For this review, take the finished solid that the model builds, in its own axes (mm). A direction names the side the tool comes from. Round coordinates to 2 decimals unless told otherwise and drop trailing zeros. Write each loop counter-clockwise with the first axis right and the second up, starting at its lowest first coordinate (ties: lowest second). Pieces come first, ordered by that corner, then holes. Notation, with made-up numbers: (16.25, 62.25) - (22.25, 62.25) arc R12 cw to (22.25, 76.25) - close; hole circle Ø6 at (-2, 77.25). An arc over 180 degrees is marked (long way). One line per item, written item: value. Start each with the question number.
Q1. Mouldability with a two-part tool opening along Y and no side actions: class faces 6 (the face through (711, 25.082, 6)), 7 (the face through (797.043, 30.166, 5.54)), 8 (the face through (712, 33.338, 4)) as +Y half, -Y half, draft (parallel to the pull), parting line (faces both ways), or undercut.
Q2. Add section B-B on x = 727.5. Write out the cut boundary in (y, z).
Q3. Add section A-A on y = -9.5. Write out the cut boundary in (x, z) (3 decimals), and give its area (3 significant figures).
Q4. Add section D-D on x = 772. Write out the cut boundary in (y, z), and give its area (3 significant figures).
Q5. Add section C-C on z = 9.5. Give the number of separate pieces and of enclosed holes in the cut face, and give its area (3 significant figures).
Q6. For probe 1 along Y at (x, z) = (793, 6.5); probe 2 along Y at (x, z) = (752, 1.5); probe 3 along X at (y, z) = (-28, 8.75), list the stretches that pass through material, from the lowest coordinate up.
Q7. Clearance check with flat-ended pins moving along their axes: pin 1 Ø0.6 at (y, z) = (-10, 1) entering from -X; pin 2 Ø2 at (x, z) = (768, 1) entering from -Y; pin 3 Ø10 at (x, y) = (772, -11) entering from -Z; pin 4 Ø0.6 at (y, z) = (7, 0.5) entering from +X (3 decimals). State where each tip first meets the part, or that it passes through.
Q8. Tool access review of faces 1 (the face through (789.37, 1, 1)), 2 (the face through (729.045, 29, 1)), 3 (the face through (784.29, -29, 5)), 4 (the face through (721.71, -23, 3)), 5 (the face through (713, -23, 7)): name each direction out of +Z, -Z, +X, -X, +Y, -Y from which nothing blocks a thin tool from reaching the whole face with its end or side.
```python
from build123d import *

# Parameters (mm, degrees)
EXTRUDE_1_DEPTH             = 8.255
EXTRUDE_2_DEPTH             = 50.165
CUT_EXTRUDE_1_DEPTH         = 50.165
EXTRUDE_3_DEPTH             = 8.255
CUT_EXTRUDE_2_DEPTH         = 8.255
CUT_EXTRUDE_3_DEPTH         = 8.255
CUT_EXTRUDE_4_DEPTH         = 55.245
CUT_EXTRUDE_5_DEPTH         = 0.635
CUT_EXTRUDE_6_DEPTH         = 46.99
SKETCH_10_W                 = 8.255
SKETCH_10_H                 = 4
EXTRUDE_4_DEPTH             = 0.635
CUT_EXTRUDE_7_DEPTH         = 2
EXTRUDE_5_DEPTH             = 8.255
SKETCH_13_W                 = 11.176
SKETCH_13_H                 = 4.318
CUT_EXTRUDE_8_DEPTH         = 3
CUT_EXTRUDE_9_DEPTH         = 12
SKETCH_15_W                 = 7.62
SKETCH_15_H                 = 31.75
CUT_EXTRUDE_10_DEPTH        = 3
HOLE_WIZARD_3_6_3_6_1_D     = 3.6
HOLE_WIZARD_3_6_3_6_1_DEPTH = 11
HOLE_WIZARD_3_6_3_6_2_D     = 3.6
HOLE_WIZARD_3_6_3_6_2_DEPTH = 11
FILLET_1_R                  = 0.635
FILLET_2_R                  = 2


with BuildPart() as part:
    # 草图1 → 凸台-拉伸1 (new body)
    with BuildSketch(Plane.XZ.offset(-25.0825)):
        with BuildLine():
            Line((729.045, 11), (729.045, 4))
            Line((729.045, 4), (721.71, 4))
            Line((721.71, 4), (718.71, 7))
            Line((718.71, 7), (715.71, 7))
            Line((715.71, 7), (715.71, 11))
            Line((715.71, 11), (705.298322179, 11))
            ThreePointArc((705.298322179, 11), (702.984819943, 5.616840019), (701.316943399, 0))
            Line((701.316943399, 0), (798.683056601, 0))
            ThreePointArc((798.683056601, 0), (797.015180057, 5.616840019), (794.701677821, 11))
            Line((794.701677821, 11), (729.045, 11))
        make_face()
    extrude(amount=-EXTRUDE_1_DEPTH)

    # 草图2 → 凸台-拉伸2 (add)
    with BuildSketch(Plane.XZ.offset(-25.0825)):
        with BuildLine():
            Line((705.298322179, 11), (715.71, 11))
            Line((715.71, 11), (715.71, 7))
            Line((715.71, 7), (718.71, 7))
            Line((718.71, 7), (721.71, 4))
            Line((721.71, 4), (792.545, 4))
            Line((792.545, 4), (792.545, 0))
            Line((792.545, 0), (701.316943399, 0))
            ThreePointArc((701.316943399, 0), (702.984819943, 5.616840019), (705.298322179, 11))
        make_face()
    extrude(amount=EXTRUDE_2_DEPTH)

    # 草图3 → 切除-拉伸1 (cut)
    with BuildSketch(Plane.XZ.offset(25.0825)):
        with BuildLine():
            Line((701.316943399, 0), (707.455, 0))
            Line((707.455, 0), (707.455, 7))
            Line((707.455, 7), (715.71, 7))
            Line((715.71, 7), (715.71, 11))
            Line((715.71, 11), (705.298322179, 11))
            ThreePointArc((705.298322179, 11), (702.984819943, 5.616840019), (701.316943399, 0))
        make_face()
    extrude(amount=-CUT_EXTRUDE_1_DEPTH, mode=Mode.SUBTRACT)

    # 草图4 → 凸台-拉伸3 (add)
    with BuildSketch(Plane.XZ.offset(25.0825)):
        with BuildLine():
            Line((705.298322179, 11), (715.71, 11))
            Line((715.71, 11), (715.71, 7))
            Line((715.71, 7), (718.71, 7))
            Line((718.71, 7), (721.71, 4))
            Line((721.71, 4), (792.545, 4))
            Line((792.545, 4), (792.545, 0))
            Line((792.545, 0), (701.316943399, 0))
            ThreePointArc((701.316943399, 0), (702.984819943, 5.616840019), (705.298322179, 11))
        make_face()
    extrude(amount=EXTRUDE_3_DEPTH)

    # 草图5 → 切除-拉伸2 (cut)
    with BuildSketch(Plane(origin=(0, 33.3375, 0), x_dir=(-1, 0, 0), z_dir=(0, 1, 0))):
        Polygon((-721.71, 4), (-715.71, 4), (-715.71, 7), (-718.71, 7), align=None)
    extrude(amount=-CUT_EXTRUDE_2_DEPTH, mode=Mode.SUBTRACT)

    # 草图6 → 切除-拉伸3 (cut)
    with BuildSketch(Plane.XZ.offset(33.3375)):
        Polygon((715.71, 0), (792.545, 0), (792.545, 4), (721.71, 4), (718.71, 7), (715.71, 7), align=None)
    extrude(amount=-CUT_EXTRUDE_3_DEPTH, mode=Mode.SUBTRACT)

    # 草图7 → 切除-拉伸4 (cut)
    with BuildSketch(Plane.ZY.offset(-729.045)):
        Polygon((0, 33.3375), (0, 24.8705), (4, 24.8705), (4, 25.0825), (11, 25.0825), (11, 33.3375), align=None)
    extrude(amount=-CUT_EXTRUDE_4_DEPTH, mode=Mode.SUBTRACT)

    # 草图8 → 切除-拉伸5 (cut)
    with BuildSketch(Plane.XZ.offset(25.0825)):
        Polygon((715.71, 0), (792.545, 0), (792.545, 4), (721.71, 4), (718.71, 7), (715.71, 7), align=None)
    extrude(amount=-CUT_EXTRUDE_5_DEPTH, mode=Mode.SUBTRACT)

    # 草图9 → 切除-拉伸6 (cut)
    with BuildSketch(Plane(origin=(0, 25.0825, 0), x_dir=(-1, 0, 0), z_dir=(0, 1, 0))):
        Polygon((-721.71, 4), (-714.44, 4), (-714.44, 0), (-707.455, 0), (-707.455, 7), (-718.71, 7), align=None)
    extrude(amount=-CUT_EXTRUDE_6_DEPTH, mode=Mode.SUBTRACT)

    # 草图10 → 凸台-拉伸4 (add)
    with BuildSketch(Plane.XZ.offset(24.4475)):
        with Locations((788.4175, 2)):
            Rectangle(SKETCH_10_W, SKETCH_10_H)
    extrude(amount=EXTRUDE_4_DEPTH)

    # 草图11 → 切除-拉伸7 (cut)
    with BuildSketch(Plane.XY.offset(4)):
        Polygon((784.29, 25.0825), (784.29, 24.8705), (729.045, 24.8705), (729.045, 33.3375), (715.71, 33.3375), (715.71, 25.0825), (714.44, 25.0825), (714.44, -21.9075), (721.71, -21.9075), (721.71, -24.4475), (784.29, -24.4475), (784.29, -25.0825), (792.545, -25.0825), (792.545, 25.0825), align=None)
    extrude(amount=-CUT_EXTRUDE_7_DEPTH, mode=Mode.SUBTRACT)

    # 草图12 → 凸台-拉伸5 (add)
    with BuildSketch(Plane.XZ.offset(25.0825)):
        with BuildLine():
            Line((798.683056601, 0), (784.29, 0))
            Line((784.29, 0), (784.29, 11))
            Line((784.29, 11), (794.701677821, 11))
            ThreePointArc((794.701677821, 11), (797.015180057, 5.616840019), (798.683056601, 0))
        make_face()
    extrude(amount=EXTRUDE_5_DEPTH)

    # 草图13 → 切除-拉伸8 (cut, through all)
    with BuildSketch(Plane.XY.offset(2)):
        with Locations((739.713, -22.2885)):
            Rectangle(SKETCH_13_W, SKETCH_13_H)
    extrude(amount=-CUT_EXTRUDE_8_DEPTH, mode=Mode.SUBTRACT)

    # 草图14 → 切除-拉伸9 (cut, through all)
    with BuildSketch(Plane(origin=(0, 0, 0), x_dir=(-1, 0, 0), z_dir=(0, 0, -1))):
        with BuildLine():
            Line((-777.963, 18.3705), (-777.963, 1.3705))
            Line((-777.963, 1.3705), (-778.963, 1.3705))
            Line((-778.963, 1.3705), (-778.963, -5.6295))
            Line((-778.963, -5.6295), (-777.963, -5.6295))
            Line((-777.963, -5.6295), (-777.963, -13.6295))
            ThreePointArc((-777.963, -13.6295), (-775.488126266, -14.654626266), (-774.463, -17.1295))
            Line((-774.463, -17.1295), (-724.463, -17.1295))
            ThreePointArc((-724.463, -17.1295), (-723.437873734, -14.654626266), (-720.963, -13.6295))
            Line((-720.963, -13.6295), (-720.963, 18.3705))
            ThreePointArc((-720.963, 18.3705), (-723.437873734, 19.395626266), (-724.463, 21.8705))
            Line((-724.463, 21.8705), (-774.463, 21.8705))
            ThreePointArc((-774.463, 21.8705), (-775.488126266, 19.395626266), (-777.963, 18.3705))
        make_face()
    extrude(amount=-CUT_EXTRUDE_9_DEPTH, mode=Mode.SUBTRACT)

    # 草图15 → 切除-拉伸10 (cut, through all)
    with BuildSketch(Plane.XY.offset(2)):
        with Locations((785.56, 0.9525)):
            Rectangle(SKETCH_15_W, SKETCH_15_H)
    extrude(amount=-CUT_EXTRUDE_10_DEPTH, mode=Mode.SUBTRACT)

    # Ø3.6 (3.6) 直径孔1
    with Locations(Plane(origin=(0, 0, 0), x_dir=(-1, 0, 0), z_dir=(0, 0, -1))):
        with Locations((-711.265, 29.5275), (-788.735, 29.5275), (-788.735, -29.5275), (-711.265, -29.5275)):
            Hole(HOLE_WIZARD_3_6_3_6_1_D / 2, depth=HOLE_WIZARD_3_6_3_6_1_DEPTH)

    # Ø3.6 (3.6) 直径孔2
    with Locations(Plane(origin=(0, 0, 0), x_dir=(-1, 0, 0), z_dir=(0, 0, -1))):
        with Locations((-720.963, -17.1295), (-720.963, 21.8705), (-777.963, 21.8705), (-777.963, -17.1295)):
            Hole(HOLE_WIZARD_3_6_3_6_2_D / 2, depth=HOLE_WIZARD_3_6_3_6_2_DEPTH)

    # 圆角1
    fillet_1_edges = [part.edges().sort_by_distance(p)[0] for p in [
        (711.5825, -25.0825, 7),
        (707.455, -23.495, 7),
        (707.455, -25.0825, 3.5),
    ]]
    fillet(fillet_1_edges, radius=FILLET_1_R)

    # 圆角2
    fillet_2_edges = [part.edges().sort_by_distance(p)[0] for p in [
        (797.015180057, -25.0825, 5.616840019),
        (702.984819943, 25.0825, 5.616840019),
        (702.984819943, -25.0825, 5.616840019),
        (797.015180057, 25.0825, 5.616840019),
    ]]
    fillet(fillet_2_edges, radius=FILLET_2_R)


solid = part.part
```
Result set:
1. face 6: undercut
1. face 7: draft
1. face 8: +Y half
2. outline: (-24.45, 0) - (-17.13, 0) - (-17.13, 2) - (-24.45, 2) - close; (21.87, 0) - (33.34, 0) - (33.34, 2) - (21.87, 2) - close
3. outline: (714.44, 0) - (720.963, 0) - (720.963, 2) - (714.44, 2) - close; (777.963, 0) - (781.75, 0) - (781.75, 2) - (777.963, 2) - close; (789.37, 0) - (792.545, 0) - (792.545, 2) - (789.37, 2) - close
3. area: 27.0 mm^2
4. outline: (-24.45, 0) - (-17.13, 0) - (-17.13, 2) - (-24.45, 2) - close; (21.87, 0) - (24.87, 0) - (24.87, 2) - (21.87, 2) - close
4. area: 20.6 mm^2
5. separate pieces: 4
5. enclosed holes: 4
5. area: 323 mm^2
6. probe 1: y = -33.34 to -25.08, 25.08 to 33.34
6. probe 2: y = -24.45 to -17.13, 21.87 to 24.87
6. probe 3: x = 704.24 to 710.31, 712.22 to 715.71, 784.29 to 787.78, 789.69 to 795.76
7. pin 1: stops at x = 714.44
7. pin 2: stops at y = -24.45
7. pin 3: passes through
7. pin 4: stops at x = 792.545
8. face 1: +Z, -Z
8. face 2: +Z, -Z, +Y
8. face 3: +Z, -Z, -Y
8. face 4: +Z, +X, +Y, -Y
8. face 5: +Z, +X, -X
